Build history of the part. All positions in model axes, mm. Face numbers are marked on the shaded views. A direction names the side the tool comes from. Coordinates: 2 decimals unless noted, no trailing zeros. Order: outer loops, then holes, each group sorted by start corner. A loop starts at its lowest first (then second) coordinate and runs counter-clockwise, first axis right, second up. Notation, with made-up numbers: (83, -15) - (138, -15) arc R22 ccw to (138, -2) - close; hole circle Ø2 at (-31, -10). An arc over 180 degrees is marked (long way). Write each question's results on one line, items separated by ' | '. Start each with the question number.
from build123d import *

# Parameters (mm, degrees)
SKETCH_1_W          = 62
SKETCH_1_H          = 25
EXTRUDE_1_DEPTH     = 30
SHELL_1_T           = -2
SKETCH_2_W          = 8
SKETCH_2_H          = 21
EXTRUDE_2_DEPTH     = 8
SKETCH_3_R          = 2
CUT_EXTRUDE_1_DEPTH = 39.951893407
SKETCH_4_R          = 6
CUT_EXTRUDE_2_DEPTH = 44.603325561
SKETCH_5_R          = 2
EXTRUDE_3_DEPTH     = 6
SKETCH_6_R          = 7
EXTRUDE_4_DEPTH     = 1
SKETCH_10_R         = 3.5
SKETCH_10_R_2       = 1.25
CUT_EXTRUDE_3_DEPTH = 74.015409333
FILLET_1_R          = 4
FILLET_2_R          = 1


with BuildPart() as part:
    # 草图1 → 凸台-拉伸1 (new body)
    with BuildSketch(Plane(origin=(0, 0, 0), x_dir=(1, 0, 0), z_dir=(0, 1, 0))):
        Rectangle(SKETCH_1_W, SKETCH_1_H)
    extrude(amount=EXTRUDE_1_DEPTH)

    # 抽壳1
    shell_1_openings = [part.faces().sort_by_distance(p)[0] for p in [
        (0, 30, 0),
    ]]
    offset(amount=SHELL_1_T, openings=shell_1_openings, kind=Kind.INTERSECTION)

    # 草图2 → 凸台-拉伸2 (add)
    with BuildSketch(Plane(origin=(0, 2, 0), x_dir=(1, 0, 0), z_dir=(0, 1, 0))):
        with Locations((-25, 0)):
            Rectangle(SKETCH_2_W, SKETCH_2_H)
        with Locations((25, 0)):
            Rectangle(SKETCH_2_W, SKETCH_2_H)
    extrude(amount=EXTRUDE_2_DEPTH)

    # 草图3 → 切除-拉伸1 (cut, through all)
    with BuildSketch(Plane(origin=(0, 10, 0), x_dir=(1, 0, 0), z_dir=(0, 1, 0))):
        with Locations(Location((25, -5, 0), (0, 0, 270))):
            Circle(SKETCH_3_R)
        with Locations(Location((25, 5, 0), (0, 0, 270))):
            Circle(SKETCH_3_R)
        with Locations(Location((-25, 5, 0), (0, 0, 90))):
            Circle(SKETCH_3_R)
        with Locations(Location((-25, -5, 0), (0, 0, 90))):
            Circle(SKETCH_3_R)
    extrude(amount=-CUT_EXTRUDE_1_DEPTH, mode=Mode.SUBTRACT)

    # 草图4 → 切除-拉伸2 (cut, through all)
    with BuildSketch(Plane(origin=(0, 2, 0), x_dir=(1, 0, 0), z_dir=(0, 1, 0))):
        with Locations(Location((-12, 0, 0), (0, 0, 270))):
            Circle(SKETCH_4_R)
    extrude(amount=-CUT_EXTRUDE_2_DEPTH, mode=Mode.SUBTRACT)

    # 草图5 → 凸台-拉伸3 (add)
    # profile 1 of 4: a face of its own
    with BuildSketch(Plane(origin=(0, 0, 0), x_dir=(1, 0, 0), z_dir=(0, 1, 0))):
        with BuildLine():
            Line((22.067619242, 18.232380758), (21, 12.5))
            Line((21, 12.5), (31, 12.5))
            Line((31, 12.5), (29.932380758, 18.232380758))
            ThreePointArc((29.932380758, 18.232380758), (26, 21.5), (22.067619242, 18.232380758))
        make_face()
        with Locations(Location((26, 17.5, 0), (0, 0, 270))):
            Circle(SKETCH_5_R, mode=Mode.SUBTRACT)
    # profile 2 of 4: a face of its own
    with BuildSketch(Plane(origin=(0, 0, 0), x_dir=(1, 0, 0), z_dir=(0, 1, 0))):
        with BuildLine():
            Line((2.067619242, 18.232380758), (1, 12.5))
            Line((1, 12.5), (11, 12.5))
            Line((11, 12.5), (9.932380758, 18.232380758))
            ThreePointArc((9.932380758, 18.232380758), (6, 21.5), (2.067619242, 18.232380758))
        make_face()
        with Locations(Location((6, 17.5, 0), (0, 0, 270))):
            Circle(SKETCH_5_R, mode=Mode.SUBTRACT)
    # profile 3 of 4: a face of its own
    with BuildSketch(Plane(origin=(0, 0, 0), x_dir=(1, 0, 0), z_dir=(0, 1, 0))):
        with BuildLine():
            Line((11, -12.5), (9.932380758, -18.232380758))
            ThreePointArc((9.932380758, -18.232380758), (6, -21.5), (2.067619242, -18.232380758))
            Line((2.067619242, -18.232380758), (1, -12.5))
            Line((1, -12.5), (11, -12.5))
        make_face()
        with Locations(Location((6, -17.5, 0), (0, 0, 90))):
            Circle(SKETCH_5_R, mode=Mode.SUBTRACT)
    # profile 4 of 4: a face of its own
    with BuildSketch(Plane(origin=(0, 0, 0), x_dir=(1, 0, 0), z_dir=(0, 1, 0))):
        with BuildLine():
            Line((31, -12.5), (29.932380758, -18.232380758))
            ThreePointArc((29.932380758, -18.232380758), (26, -21.5), (22.067619242, -18.232380758))
            Line((22.067619242, -18.232380758), (21, -12.5))
            Line((21, -12.5), (31, -12.5))
        make_face()
        with Locations(Location((26, -17.5, 0), (0, 0, 90))):
            Circle(SKETCH_5_R, mode=Mode.SUBTRACT)
    extrude(amount=EXTRUDE_3_DEPTH)

    # 草图6 → 凸台-拉伸4 (add)
    with BuildSketch(Plane(origin=(31, 0, 0), x_dir=(0, 0, -1), z_dir=(1, 0, 0))):
        with Locations((0, 20)):
            Circle(SKETCH_6_R)
    extrude(amount=EXTRUDE_4_DEPTH)

    # 草图7 → 切除-旋转1 (revolve, cut)
    with BuildSketch(Plane.XY, mode=Mode.PRIVATE) as cut_revolve_1_sk:
        Polygon((31, 27), (33, 27), (33, 25), align=None)
    revolve(cut_revolve_1_sk.sketch.rotate(Axis((32, 20, 0), (-1, 0, 0)), 90), axis=Axis((32, 20, 0), (-1, 0, 0)), mode=Mode.SUBTRACT)

    # 草图10 → 切除-拉伸3 (cut, through all)
    with BuildSketch(Plane.ZY.offset(31)):
        with Locations((0, 20)):
            Circle(SKETCH_10_R)
        with Locations((-4.949747468, 24.949747468)):
            Circle(SKETCH_10_R_2)
        with Locations((4.949747468, 24.949747468)):
            Circle(SKETCH_10_R_2)
        with Locations((4.949747468, 15.050252532)):
            Circle(SKETCH_10_R_2)
        with Locations((-4.949747468, 15.050252532)):
            Circle(SKETCH_10_R_2)
    extrude(amount=-CUT_EXTRUDE_3_DEPTH, mode=Mode.SUBTRACT)

    # 圆角1
    fillet_1_edges = [part.edges().sort_by_distance(p)[0] for p in [
        (-31, 15, 12.5),
        (-31, 15, -12.5),
    ]]
    fillet(fillet_1_edges, radius=FILLET_1_R)

    # 圆角2
    fillet_2_edges = [part.edges().sort_by_distance(p)[0] for p in [
        (29, 20, 10.5),
        (29, 20, -10.5),
        (-29, 20, -10.5),
        (-29, 20, 10.5),
    ]]
    fillet(fillet_2_edges, radius=FILLET_2_R)


solid = part.part
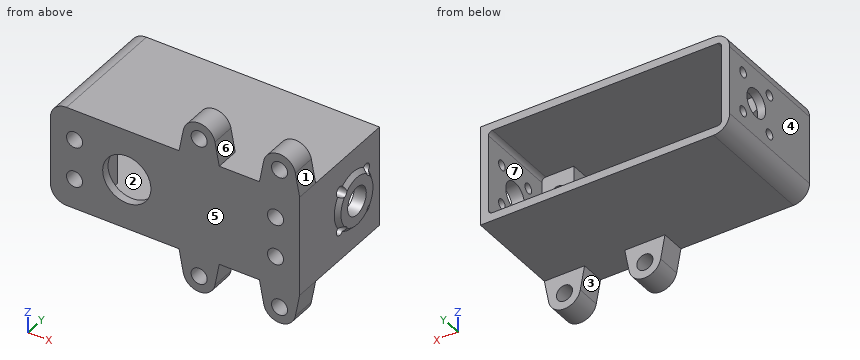
Item 1: Slice it at B-B (z = 0). Write the cut outline in (x, y), then the cut area to 3 significant figures.
Item 2: Which spindle directions (+Z, -Z, +X, -X, +Y, -Y) get a long thin tool onto all of the face, cutting with end or side? Do the marked faces 5, 6 and 7. Say none if no direction does.
Item 3: Slice it at C-C (x = 6). Write the cut outline in (y, z), then the cut area to 3 significant figures.
Item 4: Flat gauge pins, fed straight in: P1, Ø6, axis at x = 9.5, y = 6, coming from the -Z side; P2, Ø2, axis at y = 15.05, z = 4.95, coming from the -X side; P3, Ø6.5, axis at x = 6, z = -17.5, coming from the +Y side; P4, Ø10, axis at x = 19, y = 3.5, coming from the +Z side. Where does each tip first touch, or does it go through?
Item 5: Slice it at A-A (x = -12). Write the cut outline in (y, z).
Item 6: Slice it at D-D (y = 5). Count the separate pieces of the cut face and the enclosed holes in it, then the cut area to 3 significant figures.
Item 7: Pull direction X, two halves, no side cores. Call the marked faces 1, 2, 3 and 4: released by +X, released by -X, zero draft, split by the parting line, or undercut.
Item 8: Probe probe 1 along X at (y, z) = (4.5, 5); probe 2 along Z at (x, y) = (-0.5, 4); probe 3 along X at (y, z) = (2.5, 0.5). List the from-to ranges inside material, lowest first.
Resolved:
1) outline: (-31, 0) - (-18, 0) - (-18, 2) - (-21, 2) - (-21, 10) - (-29, 10) - (-29, 16.5) - (-31, 16.5) - close; (-31, 23.5) - (-29, 23.5) - (-29, 30) - (-31, 30) - close; (-6, 0) - (31, 0) - (31, 13) - (32, 14) - (32, 16.5) - (29, 16.5) - (29, 10) - (21, 10) - (21, 2) - (-6, 2) - close; (29, 23.5) - (32, 23.5) - (32, 26) - (31, 27) - (31, 30) - (29, 30) - close | area: 318 mm^2
2) face 5: +Z, -Z, +X, -X, -Y | face 6: +Z, +Y, -Y | face 7: +Y
3) outline: (0, -21.5) - (6, -21.5) - (6, -19.5) - (0, -19.5) - close; (0, -15.5) - (6, -15.5) - (6, -12.5) - (30, -12.5) - (30, -10.5) - (2, -10.5) - (2, 10.5) - (30, 10.5) - (30, 12.5) - (6, 12.5) - (6, 15.5) - (0, 15.5) - close; (0, 19.5) - (6, 19.5) - (6, 21.5) - (0, 21.5) - close | area: 222 mm^2
4) P1: z = -21.47 | P2: through | P3: y = 6 | P4: z = 20.96
5) outline: (0, -12.5) - (30, -12.5) - (30, -10.5) - (2, -10.5) - (2, -6) - (0, -6) - close; (0, 6) - (2, 6) - (2, 10.5) - (30, 10.5) - (30, 12.5) - (0, 12.5) - close
6) separate pieces: 1 | enclosed holes: 9 | area: 843 mm^2
7) face 1: released by +X | face 2: undercut | face 3: undercut | face 4: released by -X
8) probe 1: -31 to -27, -23 to -21, 21 to 23, 27 to 31 | probe 2: -12.5 to -10.5, 10.5 to 12.5 | probe 3: -31 to -21, 21 to 31
